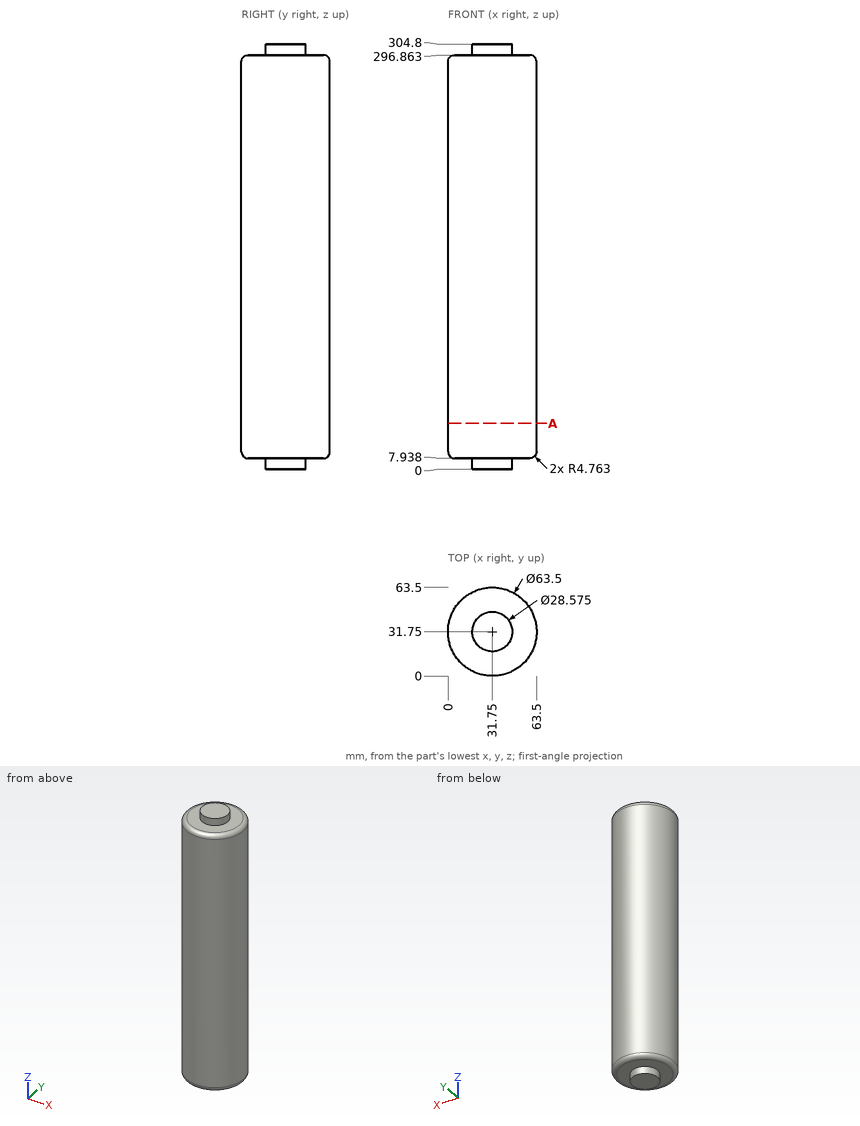
Drawing for the job (mm, zero at the part's lowest x, y, z). Round coordinates to 2 decimals unless told otherwise and drop trailing zeros. Write each loop counter-clockwise with the first axis right and the second up, starting at its lowest first coordinate (ties: lowest second). Pieces come first, ordered by that corner, then holes.
Item 1: Band-saw the part on A-A on z = 33. Write the cut outline in (x, y).
Filled in:
outline: circle Ø63.5 at (31.75, 31.75)
Item 2: Drill centre lines: L1, parallel to Z at x = 4.5, y = 32 (1 decimal); L2, parallel to Y at x = 31, z = 227.5. Where is each one in solid material? Low to high.
Filled in:
L1: z = 7.9 to 296.9
L2: y = 0.01 to 63.49
Item 3: Drop flat-ended pins along their axis: pin 1 Ø1 at (y, z) = (7, 103) entering from +X (1 decimal); pin 2 Ø8 at (x, z) = (19, 218) entering from +Y; pin 3 Ø8 at (y, z) = (52, 248.5) entering from -X (1 decimal). Give the stop position or say it passes through.
Filled in:
pin 1: stops at x = 52.2
pin 2: stops at y = 62.27
pin 3: stops at x = 4.5
